```python
from build123d import *

# Parameters (mm, degrees)
SKETCH1_W                = 264
SKETCH1_H                = 60
BOSS_EXTRUDE1_DEPTH      = 3
BOSS_EXTRUDE2_DEPTH      = 125
BOSS_EXTRUDE2_DEPTH_BACK = 125
FILLET1_R                = 1


with BuildPart() as part:
    # Sketch1 → Boss-Extrude1 (new body)
    with BuildSketch(Plane.XY):
        Rectangle(SKETCH1_W, SKETCH1_H)
    extrude(amount=BOSS_EXTRUDE1_DEPTH)

    # Sketch2 → Boss-Extrude2 (add, two sides)
    with BuildSketch(Plane(origin=(0, 0, 0), x_dir=(0, 0, -1), z_dir=(1, 0, 0))) as boss_extrude2_sk:
        Polygon((0, 28), (4.73, 28), (11.605935411, -28), (0, -28), align=None)
    extrude(amount=BOSS_EXTRUDE2_DEPTH)
    extrude(boss_extrude2_sk.sketch, amount=-BOSS_EXTRUDE2_DEPTH_BACK)

    # Fillet1
    fillet1_edges = [part.edges().sort_by_distance(p)[0] for p in [
        (125, 28, -2.365),
        (125, -28, -5.802967705),
        (-125, 28, -2.365),
        (-125, -28, -5.802967705),
        (-132, 30, 1.5),
        (132, 30, 1.5),
        (132, -30, 1.5),
        (-132, -30, 1.5),
    ]]
    fillet(fillet1_edges, radius=FILLET1_R)


solid = part.part
```
Verification items for the finished model (mm, model axes). A direction names the side the tool comes from. Round coordinates to 2 decimals unless told otherwise and drop trailing zeros. Loops run counter-clockwise (first coordinate to the right, second up) from the corner with the lowest first, then second, coordinate; pieces in that order, holes last. Notation, with made-up numbers: (78, -8.75) -> (124, -8.75) arc R22 cw to (124, 29.25) -> close; hole circle Ø6 at (6.25, 83). An arc over 180 degrees is marked (long way). Answer as a JSON object with one key per item and string values.
Q1. Scan lines: line 1 (X direction, y = 19.5, z = -3); line 2 (Y direction, x = -115, z = -3.75); line 3 (Z direction, x = 84.5, y = 11.5). Record each from-to range of solid material in increasing order. Write a range as from..to.
Data:
{"line 1": "x = -125..125", "line 2": "y = -28..28", "line 3": "z = -6.76..3"}
Q2. Section check C-C (z = -8.5). Record the boundary of the cut face in (x, y), then the cut area to 3 significant figures.
Data:
{"outline": "(-125, -27) arc R1 ccw to (-124, -28) -> (124, -28) arc R1 ccw to (125, -27) -> (125, -2.7) -> (-125, -2.7) -> close", "area": "6,320 mm2"}
Q3. Access from +Z, -Z, +X, -X, +Y, -Y to the whole of each face (thin tool, end or side, straight path). Record for faces 1 (the flat face through (2, 28, -2)), 2 (the flat face through (125, -6, -5)), 3 (the flat face through (-2, -28, -6)), 4 (the flat face through (-125, -6, -5)), 5 (the flat face through (-1, 29, 0)).
Data:
{"face 1": "-Z, +X, -X, +Y", "face 2": "-Z, +X, +Y, -Y", "face 3": "-Z, +X, -X, -Y", "face 4": "-Z, -X, +Y, -Y", "face 5": "-Z"}
Q4. Go/stop test with flat-tipped pins: P1, Ø5.5, axis at y = 9.5, z = -7.5, coming from the +X side; P2, Ø5.5, axis at y = -8, z = -4, coming from the -X side; P3, Ø3, axis at x = -67.5, z = -8.5, coming from the -Y side; P4, Ø1.5, axis at y = -2.5, z = -9.5, coming from the -X side. Record where each tip stops, or that it passes through.
Data:
{"P1": "stops at x = 125", "P2": "stops at x = -125", "P3": "stops at y = -28", "P4": "passes through"}
Q5. Section check B-B (x = 35). Record the boundary of the cut face in (y, z).
Data:
{"outline": "(-30, 0) -> (-28, 0) -> (-28, -11.61) -> (28, -4.73) -> (28, 0) -> (30, 0) -> (30, 3) -> (-30, 3) -> close"}
Q6. Section check A-A (y = -11.5). Record the boundary of the cut face in (x, z), then the cut area to 3 significant figures.
Data:
{"outline": "(-132, 0) -> (-125, 0) -> (-125, -9.58) -> (125, -9.58) -> (125, 0) -> (132, 0) -> (132, 3) -> (-132, 3) -> close", "area": "3,190 mm2"}
